Check sheet for the modelled part. Datum: model origin and axes. Units: mm. A direction names the side the tool comes from. Round coordinates to 2 decimals unless told otherwise and drop trailing zeros. Write each loop counter-clockwise with the first axis right and the second up, starting at its lowest first coordinate (ties: lowest second). Pieces come first, ordered by that corner, then holes. Notation, with made-up numbers: (43, 15.5) -> (91, 15.5) arc R8 ccw to (91, 25.5) -> close; hole circle Ø9 at (-2.75, 40). An arc over 180 degrees is marked (long way). Write item = value, one per line.
from build123d import *

# Parameters (mm, degrees)
F0_R      = 17.4625
F0_R_2    = 12.7
F0_R_3    = 2.0931181944
F0_R_4    = 5.588
F0_R_5    = 2.413
F1_DEPTH  = 3.175
F2_R      = 3.9963045726
F2_R_2    = 1.9205832971
F3_DEPTH  = 1.27
F4_R      = 1.8414609102
F5_DEPTH  = 1.27
F6_R      = 3.175
F7_DEPTH  = 7.62
F8_R      = 0.3211313055
F9_DEPTH  = 0.254
F10_R     = 17.4625
F10_R_2   = 13.2761533165
F11_DEPTH = 1.27
F12_R     = 17.4625
F12_R_2   = 13.1551445167
F13_DEPTH = 1.27
F14_R     = 17.4625
F14_R_2   = 15.2967108996
F15_DEPTH = 1.016


with BuildPart() as f1:
    # F0 (on Front) → F1 (new body)
    with BuildSketch(Plane.XZ):
        Circle(F0_R)
        Circle(F0_R_2, mode=Mode.SUBTRACT)
        Circle(F0_R_2)
        with Locations((-6.2330407914, -6.2330407914)):
            Circle(F0_R_3, mode=Mode.SUBTRACT)
        with Locations((0, -8.8148508221)):
            Circle(F0_R_3, mode=Mode.SUBTRACT)
        with Locations((6.2330407914, -6.2330407914)):
            Circle(F0_R_3, mode=Mode.SUBTRACT)
        with Locations((-8.8148508221, 0)):
            Circle(F0_R_3, mode=Mode.SUBTRACT)
        with Locations((-6.2330407914, 6.2330407914)):
            Circle(F0_R_3, mode=Mode.SUBTRACT)
        Circle(F0_R_4, mode=Mode.SUBTRACT)
        with Locations((6.2330407914, 6.2330407914)):
            Circle(F0_R_3, mode=Mode.SUBTRACT)
        with Locations((8.8148508221, 0)):
            Circle(F0_R_3, mode=Mode.SUBTRACT)
        with Locations((0, 8.8148508221)):
            Circle(F0_R_3, mode=Mode.SUBTRACT)
        Circle(F0_R_4)
        Circle(F0_R_5, mode=Mode.SUBTRACT)
        Circle(F0_R_5)
    extrude(amount=F1_DEPTH)

    # F2 (on face) → F3 (join)
    with BuildSketch(Plane.XZ.offset(3.175)):
        Circle(F2_R)
        Circle(F2_R_2, mode=Mode.SUBTRACT)
        Circle(F2_R_2)
    extrude(amount=F3_DEPTH)

    # F4 (on face) → F5 (join)
    with BuildSketch(Plane.XZ.offset(4.445)):
        Circle(F4_R)
    extrude(amount=F5_DEPTH)

    # F6 (on face) → F7 (join)
    with BuildSketch(Plane(origin=(0, 0, 0), x_dir=(-1, 0, 0), z_dir=(0, 1, 0))):
        Circle(F6_R)
    extrude(amount=F7_DEPTH)

    # F8 (on face) → F9 (join)
    with BuildSketch(Plane.XZ.offset(4.445)):
        with Locations((0, 2.7205995284)):
            Circle(F8_R)
        with Locations((-1.9237543754, 1.9237543754)):
            Circle(F8_R)
        with Locations((-2.7205995284, 0)):
            Circle(F8_R)
        with Locations((-1.9237543754, -1.9237543754)):
            Circle(F8_R)
        with Locations((0, -2.7205995284)):
            Circle(F8_R)
        with Locations((1.9237543754, -1.9237543754)):
            Circle(F8_R)
        with Locations((2.7205995284, 0)):
            Circle(F8_R)
        with Locations((1.9237543754, 1.9237543754)):
            Circle(F8_R)
    extrude(amount=F9_DEPTH)

    # F10 (on face) → F11 (join)
    with BuildSketch(Plane.XZ.offset(3.175)):
        Circle(F10_R)
        Circle(F10_R_2, mode=Mode.SUBTRACT)
    extrude(amount=F11_DEPTH)

    # F12 (on face) → F13 (join)
    with BuildSketch(Plane(origin=(0, 0, 0), x_dir=(-1, 0, 0), z_dir=(0, 1, 0))):
        Circle(F12_R)
        Circle(F12_R_2, mode=Mode.SUBTRACT)
    extrude(amount=F13_DEPTH)

    # F14 (on face) → F15 (join)
    with BuildSketch(Plane.XZ.offset(4.445)):
        Circle(F14_R)
        Circle(F14_R_2, mode=Mode.SUBTRACT)
    extrude(amount=F15_DEPTH)


solid = f1.part
(1) Sectioned sample at D-D on x = -11.5. Enter the section's corners in (y, z) (3 decimals), then the cut area to 3 significant figures.
Worked answers:
outline = (-5.461, -13.141) -> (1.27, -13.141) -> (1.27, -6.388) -> (0, -6.388) -> (0, 6.388) -> (1.27, 6.388) -> (1.27, 13.141) -> (-5.461, 13.141) -> (-5.461, 10.087) -> (-4.445, 10.087) -> (-4.445, 6.634) -> (-3.175, 6.634) -> (-3.175, -6.634) -> (-4.445, -6.634) -> (-4.445, -10.087) -> (-5.461, -10.087) -> close
area = 123 mm²
(2) Sectioned sample at A-A on z = -5.5. Enter the section's corners in (x, y) (3 decimals), then the cut area to 3 significant figures.
Worked answers:
outline = (-16.574, -5.461) -> (-14.274, -5.461) -> (-14.274, -4.445) -> (-12.083, -4.445) -> (-12.083, -3.175) -> (-8.194, -3.175) -> (-8.194, 0) -> (-11.95, 0) -> (-11.95, 1.27) -> (-16.574, 1.27) -> close; (-4.272, -3.175) -> (4.272, -3.175) -> (4.272, 0) -> (-4.272, 0) -> close; (8.194, -3.175) -> (12.083, -3.175) -> (12.083, -4.445) -> (14.274, -4.445) -> (14.274, -5.461) -> (16.574, -5.461) -> (16.574, 1.27) -> (11.95, 1.27) -> (11.95, 0) -> (8.194, 0) -> close
area = 108 mm²
(3) Release check for a two-part mould opening along Z. For faces 1 (the flat face through (0, -5.715, 0)), 2 (the flat face through (3, -3.175, 3)) record: pulls with the +Z half, pulls with the -Z half, needs draft (parallel to the pull), parting line crosses it, or undercut.
Worked answers:
face_1 = needs draft
face_2 = undercut
(4) Material ranges on L1, parallel to Z at x = 0, y = -2; L2, parallel to Z at x = 0, y = -4.65; L3, parallel to X at y = -1.5, z = -0.5, recorded low to high. Write a range as [from, to].
Worked answers:
L1 = [-17.46, -10.91], [-6.72, 6.72], [10.91, 17.46]
L2 = [-17.46, -15.3], [-3.04, -2.4], [-1.84, 1.84], [2.4, 3.04], [15.3, 17.46]
L3 = [-17.46, -10.85], [-6.78, 6.78], [10.85, 17.46]
(5) Sectioned sample at B-B on y = -2.75. Count the separate pieces of the cut face and the enclosed holes in it, then the cut area to 3 significant figures.
Worked answers:
separate_pieces = 1
enclosed_holes = 8
area = 848 mm²
(6) Go/stop test with flat-tipped pins: P1, Ø3, axis at x = -11.5, y = -1, coming from the -Z side; P2, Ø3, axis at y = 5.5, z = -6, coming from the +X side; P3, Ø6.5, axis at x = 0, z = 8.81, coming from the -Y side (3 decimals); P4, Ø0.5, axis at x = -2, z = 2, coming from the -Y side. Record where each tip stops, or that it passes through.
Worked answers:
P1 = -14.32
P2 = through
P3 = -3.175
P4 = -4.7
(7) Sectioned sample at C-C on z = -10. Enter the section's corners in (x, y) (3 decimals).
Worked answers:
outline = (-14.316, -5.461) -> (-11.575, -5.461) -> (-11.575, -4.445) -> (-8.732, -4.445) -> (-8.732, -3.175) -> (-1.725, -3.175) -> (-1.725, 0) -> (-8.547, 0) -> (-8.547, 1.27) -> (-14.316, 1.27) -> close; (1.725, -3.175) -> (8.732, -3.175) -> (8.732, -4.445) -> (11.575, -4.445) -> (11.575, -5.461) -> (14.316, -5.461) -> (14.316, 1.27) -> (8.547, 1.27) -> (8.547, 0) -> (1.725, 0) -> close
(8) Access from +Z, -Z, +X, -X, +Y, -Y to the whole of each face (thin tool, end or side, straight path). Record for faces 3 (the flat face through (3, 0, -3)), 4 (the cylindrical face through (-0.87, -3.8, -3.9)), 5 (the cylindrical face through (7.15, -1.57, -1.27)).
Worked answers:
face_3 = +Y
face_4 = -Y
face_5 = +Y, -Y
